from build123d import *

# Parameters (mm, degrees)
F1_DEPTH      = 4
F2_R          = 4.345587
F3_DEPTH      = 2
F3_DEPTH_BACK = 6
F5_DEPTH      = 25
F6_R          = 4.04816
F7_DEPTH      = 2
F8_R          = 2.39956
F9_DEPTH      = 0.4
F10_R         = 1.472917
F11_DEPTH     = 25
F12_R         = 3.987391
F13_DEPTH     = 5
F14_R         = 2.881593
F15_DEPTH     = 1
F16_R         = 1.676449
F17_DEPTH     = 25
F18_SIZE      = 0.5


with BuildPart() as f1:
    # F0 (on Front) → F1 (new body)
    with BuildSketch(Plane.XZ):
        with BuildLine():
            Line((19.393065, -2.246393), (4.379365, 25.005329))
            ThreePointArc((4.379365, 25.005329), (0, 27.59262), (-4.379365, 25.005329))
            Line((-4.379365, 25.005329), (-19.393065, -2.246393))
            ThreePointArc((-19.393065, -2.246393), (-17.81974, -7.680052), (-12.386081, -6.106727))
            Line((-12.386081, -6.106727), (-3.503492, 10.01627))
            ThreePointArc((-3.503492, 10.01627), (0, 12.086103), (3.503492, 10.01627))
            Line((3.503492, 10.01627), (12.386081, -6.106727))
            ThreePointArc((12.386081, -6.106727), (17.81974, -7.680052), (19.393065, -2.246393))
        make_face()
    extrude(amount=F1_DEPTH)

    # F2 (on face) → F3 (join, two sides)
    with BuildSketch(Plane.XZ.offset(4)) as f3_sk:
        with Locations((0, 21.446018)):
            Circle(F2_R)
    extrude(amount=F3_DEPTH)
    extrude(f3_sk.sketch, amount=-F3_DEPTH_BACK)

    # F4 (on face) → F5 (cut)
    with BuildSketch(Plane.XZ.offset(6)):
        Polygon((-1.571178, 18.890357), (1.427678, 18.807508), (2.998856, 21.363168), (1.571178, 24.001678), (-1.427678, 24.084528), (-2.998856, 21.528867), align=None)
    extrude(amount=-F5_DEPTH, mode=Mode.SUBTRACT)

    # F6 (on face) → F7 (join)
    with BuildSketch(Plane.XZ.offset(4)):
        with Locations((-15.889573, -4.17656)):
            Circle(F6_R)
    extrude(amount=F7_DEPTH)

    # F8 (on face) → F9 (cut)
    with BuildSketch(Plane.XZ.offset(6)):
        with Locations((-15.889573, -4.17656)):
            Circle(F8_R)
    extrude(amount=-F9_DEPTH, mode=Mode.SUBTRACT)

    # F10 (on face) → F11 (cut)
    with BuildSketch(Plane.XZ.offset(5.6)):
        with Locations((-15.889573, -4.17656)):
            Circle(F10_R)
    extrude(amount=-F11_DEPTH, mode=Mode.SUBTRACT)

    # F12 (on face) → F13 (join)
    with BuildSketch(Plane.XZ.offset(4)):
        with Locations((15.889573, -4.17656)):
            Circle(F12_R)
    extrude(amount=F13_DEPTH)

    # F14 (on face) → F15 (cut)
    with BuildSketch(Plane.XZ.offset(9)):
        with Locations((15.889573, -4.17656)):
            Circle(F14_R)
    extrude(amount=-F15_DEPTH, mode=Mode.SUBTRACT)

    # F16 (on face) → F17 (cut)
    with BuildSketch(Plane.XZ.offset(8)):
        with Locations((15.889573, -4.17656)):
            Circle(F16_R)
    extrude(amount=-F17_DEPTH, mode=Mode.SUBTRACT)

    # F18
    f18_edges = [f1.edges().sort_by_distance(p)[0] for p in [
        (11.902182, -9, -4.17656),
    ]]
    chamfer(f18_edges, length=F18_SIZE)


solid = f1.part
Work out the finished part from the listing and answer in its coordinate system (mm). A direction names the side the tool comes from. Give positions to 0.01 mm unless a question says otherwise; leave off trailing zeros. Order: outer loops, then holes, each group sorted by start corner. A loop starts at its lowest first (then second) coordinate and runs counter-clockwise, first axis right, second up. Notation, with made-up numbers: (69.5, 55) -> (124.5, 55) arc R19 ccw to (124.5, 82) -> close; hole circle Ø6 at (49.25, 12). An arc over 180 degrees is marked (long way). Answer as a JSON object with one key per item and string values. Group by question number.
1. Section B-B on y = 0.75 is taken. Determine the outline of the cut face in (x, z).
2. Flat-ended cylindrical pins translate along their axes: pin 1 Ø1.5 at (y, z) = (-6, 9.5) entering from +X; pin 2 Ø2.5 at (x, z) = (-14.5, -5.5) entering from -Y; pin 3 Ø3.5 at (x, z) = (-15.89, -4.18) entering from -Y; pin 4 Ø6 at (y, z) = (-4, 10) entering from +X. Find the tip coordinate at first contact, or state that the pin passes through.
3. Section A-A on x = 0 is taken. Determine the outline of the cut face in (y, z), plus the area to 3 significant figures.
4. Consider line 1 along X through (y, z) = (-2.5, 5); line 2 along Z through (x, y) = (1.5, -3); line 3 along Y through (x, z) = (-8, 18). Determine where each line is inside the solid, lowest interval first. Write a range as [from, to].
5. A tool of negligible diameter and unlimited length cuts with its end or side. For faces 1 (the cylindrical face through (-0.566, -4.986, 25.755)), 2 (the flat face through (-2.202, -2.056, 22.825)), 3 (the cylindrical face through (-17.896, -1.972, -7.637)), from which of +Z, -Z, +X, -X, +Y, -Y can it reach the whole face along a straight path? Write none if from no direction.
6. Section D-D on y = -1.75 is taken. Determine the outline of the cut face in (x, z).
7. Section C-C on z = 1 is taken. Determine the outline of the cut face in (x, y).
Result sheet:
{
 "1": {"outline": "circle Ø8.69 at (0, 21.45); hole (-3, 21.53) -> (-1.57, 18.89) -> (1.43, 18.81) -> (3, 21.36) -> (1.57, 24) -> (-1.43, 24.08) -> close"},
 "2": {"pin 1": "passes through", "pin 2": "stops at y = -6", "pin 3": "stops at y = -5.6", "pin 4": "stops at x = 14.3"},
 "3": {"outline": "(-6, 17.1) -> (-4, 17.1) -> (-4, 12.09) -> (0, 12.09) -> (0, 17.1) -> (2, 17.1) -> (2, 18.85) -> (-6, 18.85) -> close; (-6, 24.05) -> (2, 24.05) -> (2, 25.79) -> (0, 25.79) -> (0, 27.59) -> (-4, 27.59) -> (-4, 25.79) -> (-6, 25.79) -> close", "area": "55.2 mm^2"},
 "4": {"line 1": "x = [-15.4, -6.27], [6.27, 15.4]", "line 2": "z = [11.79, 18.93], [24, 27.36]", "line 3": "y = [-4, 0]"},
 "5": {"face 1": "-Y", "face 2": "+Y, -Y", "face 3": "+Y"},
 "6": {"outline": "(-19.39, -2.25) arc R4 ccw to (-12.39, -6.11) -> (-3.5, 10.02) arc R4 cw to (3.5, 10.02) -> (12.39, -6.11) arc R4 ccw to (19.39, -2.25) -> (4.38, 25.01) arc R5 ccw to (-4.38, 25.01) -> close; hole circle Ø2.95 at (-15.89, -4.18); hole (-3, 21.53) -> (-1.57, 18.89) -> (1.43, 18.81) -> (3, 21.36) -> (1.57, 24) -> (-1.43, 24.08) -> close; hole circle Ø3.35 at (15.89, -4.18)"},
 "7": {"outline": "(-17.6, -4) -> (-8.47, -4) -> (-8.47, 0) -> (-17.6, 0) -> close; (8.47, -4) -> (17.6, -4) -> (17.6, 0) -> (8.47, 0) -> close"}
}
